from build123d import *

# Parameters (mm, degrees)
F0_R     = 2
F1_DEPTH = 3


with BuildPart() as f1:
    # F0 (on Top) → F1 (new body)
    with BuildSketch(Plane.XY):
        with BuildLine():
            Line((-40, -33), (40, -33))
            ThreePointArc((40, -33), (50.606602, -28.606602), (55, -18))
            Line((55, -18), (55, 18))
            ThreePointArc((55, 18), (50.606602, 28.606602), (40, 33))
            Line((40, 33), (-40, 33))
            ThreePointArc((-40, 33), (-50.606602, 28.606602), (-55, 18))
            Line((-55, 18), (-55, -18))
            ThreePointArc((-55, -18), (-50.606602, -28.606602), (-40, -33))
        make_face()
        with Locations((-43.45962, -21.612271)):
            Circle(F0_R, mode=Mode.SUBTRACT)
        with Locations((0, -23)):
            Circle(F0_R, mode=Mode.SUBTRACT)
        with Locations((43.45962, -21.612271)):
            Circle(F0_R, mode=Mode.SUBTRACT)
        with Locations((-43.45962, 21.612271)):
            Circle(F0_R, mode=Mode.SUBTRACT)
        with BuildLine():
            ThreePointArc((-36, 4), (-32.571068, 11.278175), (-25, 14))
            Line((-25, 14), (25, 14))
            ThreePointArc((25, 14), (32.571068, 11.278175), (36, 4))
            Line((36, 4), (36, -2))
            ThreePointArc((36, -2), (32.778175, -9.778175), (25, -13))
            Line((25, -13), (-25, -13))
            ThreePointArc((-25, -13), (-32.778175, -9.778175), (-36, -2))
            Line((-36, -2), (-36, 4))
        make_face(mode=Mode.SUBTRACT)
        with Locations((0, 23)):
            Circle(F0_R, mode=Mode.SUBTRACT)
        with Locations((43.45962, 21.612271)):
            Circle(F0_R, mode=Mode.SUBTRACT)
    extrude(amount=F1_DEPTH)


solid = f1.part
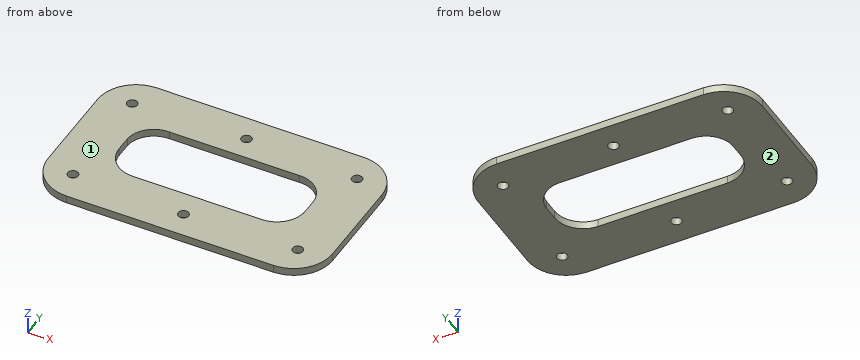
Design review of the part built by this model. Coordinates are the model's own, in mm. Face numbers are marked on the shaded views. Coordinates: 2 decimals unless noted, no trailing zeros. Order: outer loops, then holes, each group sorted by start corner. A loop starts at its lowest first (then second) coordinate and runs counter-clockwise, first axis right, second up. Notation, with made-up numbers: (28.25, 24) -> (61.25, 24) arc R15 cw to (61.25, 37) -> close; hole circle Ø3 at (-21.5, 68.25). An arc over 180 degrees is marked (long way). One line per item, written item: value.
1) We need section B-B, the plane y = -0.5. Give the boundary of the cut face in (x, z).
Output values:
outline: (-55, 0) -> (-36, 0) -> (-36, 3) -> (-55, 3) -> close; (36, 0) -> (55, 0) -> (55, 3) -> (36, 3) -> close
2) We need section C-C, the plane x = 0. Give the boundary of the cut face in (y, z).
Output values:
outline: (-33, 0) -> (-25, 0) -> (-25, 3) -> (-33, 3) -> close; (-21, 0) -> (-13, 0) -> (-13, 3) -> (-21, 3) -> close; (14, 0) -> (21, 0) -> (21, 3) -> (14, 3) -> close; (25, 0) -> (33, 0) -> (33, 3) -> (25, 3) -> close
3) To check wall thickness, follow probe 1 along Y at (x, z) = (0, 1.2); probe 2 along Y at (x, z) = (13, 1.2); probe 3 along X at (y, z) = (1.5, 2.75). State the ranges of each line that lie inside material, in increasing order. Write a range as [from, to].
Output values:
probe 1: y = [-33, -25], [-21, -13], [14, 21], [25, 33]
probe 2: y = [-33, -13], [14, 33]
probe 3: x = [-55, -36], [36, 55]
4) Draft analysis for pull direction Z (two halves, no side actions). For the marked faces 1 and 2, state which applies: +Z half, -Z half, draft (parallel to the pull), parting line (faces both ways), or undercut.
Output values:
face 1: +Z half
face 2: -Z half
5) We need section A-A, the plane x = 12.5. Give the boundary of the cut face in (y, z).
Output values:
outline: (-33, 0) -> (-13, 0) -> (-13, 3) -> (-33, 3) -> close; (14, 0) -> (33, 0) -> (33, 3) -> (14, 3) -> close
6) We need section D-D, the plane z = 2.5. Give the boundary of the cut face in (x, y).
Output values:
outline: (-55, -18) arc R15 ccw to (-40, -33) -> (40, -33) arc R15 ccw to (55, -18) -> (55, 18) arc R15 ccw to (40, 33) -> (-40, 33) arc R15 ccw to (-55, 18) -> close; hole circle Ø4 at (-43.46, -21.61); hole circle Ø4 at (-43.46, 21.61); hole (-36, -2) arc R11 ccw to (-25, -13) -> (25, -13) arc R11 ccw to (36, -2) -> (36, 4) arc R10.51 ccw to (25, 14) -> (-25, 14) arc R10.51 ccw to (-36, 4) -> close; hole circle Ø4 at (0, -23); hole circle Ø4 at (0, 23); hole circle Ø4 at (43.46, -21.61); hole circle Ø4 at (43.46, 21.61)
